```python
from build123d import *

# Parameters (mm, degrees)
F1_DEPTH = 12.7
F3_DEPTH = 25.401
F5_DEPTH = 25.4


with BuildPart() as f1:
    # F0 (on Front) → F1 (new body, symmetric)
    with BuildSketch(Plane.XZ):
        with BuildLine():
            Line((76.2, -76.2), (76.2, 0))
            Line((76.2, 0), (76.2, 76.2))
            Line((76.2, 76.2), (54.9515881949, 76.2))
            ThreePointArc((54.9515881949, 76.2), (49.567872747, 74.095124986), (47.0394765128, 68.8968461044))
            Line((47.0394765128, 68.8968461044), (44.6467865895, 39.0531538956))
            ThreePointArc((44.6467865895, 39.0531538956), (42.1183903553, 33.854875014), (36.7346749074, 31.75))
            Line((36.7346749074, 31.75), (-76.2, 31.75))
            Line((-76.2, 31.75), (-76.2, 0))
            Line((-76.2, 0), (-76.2, -31.75))
            Line((-76.2, -31.75), (36.7346749074, -31.75))
            ThreePointArc((36.7346749074, -31.75), (42.1183903553, -33.854875014), (44.6467865895, -39.0531538956))
            Line((44.6467865895, -39.0531538956), (47.0394765128, -68.8968461044))
            ThreePointArc((47.0394765128, -68.8968461044), (49.567872747, -74.095124986), (54.9515881949, -76.2))
            Line((54.9515881949, -76.2), (76.2, -76.2))
        make_face()
    extrude(amount=F1_DEPTH, both=True)

    # F2 (on face) → F3 (cut, through all)
    with BuildSketch(Plane.XZ.offset(12.7)):
        with BuildLine():
            ThreePointArc((-65.0875, 0), (-67.4123399243, 5.6126600757), (-73.025, 7.9375))
            Line((-73.025, 7.9375), (-76.2, 7.9375))
            Line((-76.2, 7.9375), (-76.2, -7.9375))
            Line((-76.2, -7.9375), (-73.025, -7.9375))
            ThreePointArc((-73.025, -7.9375), (-67.4123399243, -5.6126600757), (-65.0875, 0))
        make_face()
    extrude(amount=-F3_DEPTH, mode=Mode.SUBTRACT)

    # F4 (on face) → F5 (cut)
    with BuildSketch(Plane.XZ.offset(12.7)):
        with BuildLine():
            ThreePointArc((-25.4, -12.7), (-25.4475770151, -11.9241362755), (-25.5895951241, -11.159898781))
            ThreePointArc((-25.5895951241, -11.159898781), (-33.290101219, -6.5395951241), (-37.9104048759, -14.240101219))
            ThreePointArc((-37.9104048759, -14.240101219), (-30.9741362755, -19.0024229849), (-25.4, -12.7))
        make_face()
        with BuildLine():
            ThreePointArc((-31.9395951241, 14.240101219), (-31.7975770151, 13.4758637245), (-31.75, 12.7))
            ThreePointArc((-31.75, 12.7), (-37.3241362755, 6.3975770151), (-44.2604048759, 11.159898781))
            Line((-44.2604048759, 11.159898781), (-37.9104048759, -14.240101219))
            ThreePointArc((-37.9104048759, -14.240101219), (-33.290101219, -6.5395951241), (-25.5895951241, -11.159898781))
            Line((-25.5895951241, -11.159898781), (-31.9395951241, 14.240101219))
        make_face()
        with BuildLine():
            ThreePointArc((-44.2604048759, 11.159898781), (-37.3241362755, 6.3975770151), (-31.75, 12.7))
            ThreePointArc((-31.75, 12.7), (-31.7975770151, 13.4758637245), (-31.9395951241, 14.240101219))
            ThreePointArc((-31.9395951241, 14.240101219), (-39.640101219, 18.8604048759), (-44.2604048759, 11.159898781))
        make_face()
        with BuildLine():
            Line((-55.5874992575, -31.75), (-55.5874992575, -24.8370918305))
            ThreePointArc((-55.5874992575, -24.8370918305), (-62.0395651932, -19.0512714315), (-68.2549589201, -25.0906218393))
            Line((-68.2549589201, -25.0906218393), (-68.2549589201, -31.75))
            Line((-68.2549589201, -31.75), (-55.5874992575, -31.75))
        make_face()
    extrude(amount=-F5_DEPTH, mode=Mode.SUBTRACT)


solid = f1.part
```
Input: part model. Units: mm. Frame: model coordinates. A direction names the side the tool comes from. Coordinates: 2 decimals unless noted, no trailing zeros. Write each loop counter-clockwise with the first axis right and the second up, starting at its lowest first coordinate (ties: lowest second). Pieces come first, ordered by that corner, then holes. Notation, with made-up numbers: (-12, 35) -> (8, 35) arc R28 cw to (8, 73) -> close; hole circle Ø2 at (18, 66). An arc over 180 degrees is marked (long way). Answer as a JSON object with one key per item and string values.
1. Section B-B on x = 24. Return the cut outline in (y, z).
Result set:
{"outline": "(-12.7, -31.75) -> (12.7, -31.75) -> (12.7, 31.75) -> (-12.7, 31.75) -> close"}
2. Material intervals for line 1 (X direction, y = 1, z = -28.5); line 2 (Z direction, x = 16.5, y = 4.25); line 3 (X direction, y = 4.75, z = 6), sorted ascending. Write a range as from..to.
Result set:
{"line 1": "x = -76.2..-68.25, -55.59..76.2", "line 2": "z = -31.75..31.75", "line 3": "x = -67.83..-42.97, -29.88..76.2"}
3. Mould query, pull axis X, two halves, no side actions, for faces 6 (the face through (16, -12.7, 1)), 7 (the face through (-55.587, 0, -28)), 8 (the face through (42.18, -0.18, 33.91)). Classes: released by +X, released by -X, zero draft, split by the parting line, or undercut.
Result set:
{"face 6": "zero draft", "face 7": "undercut", "face 8": "released by -X"}
4. Access query for faces 1 (the face through (-76.2, 0, 20)), 2 (the face through (-68.255, 0, -28)), 3 (the face through (-10, 0, -31.75)), 4 (the face through (-41.13, -0.18, -1.36)), 5 (the face through (-19, 0, 31.75)). Directions: +Z, -Z, +X, -X, +Y, -Y. A direction counts if a zero-diameter tool reaches every point of the face in a straight line with its end or side. Return the directions, or none.
Result set:
{"face 1": "+Z, -Z, -X, +Y, -Y", "face 2": "-Z, +Y, -Y", "face 3": "-Z, -X, +Y, -Y", "face 4": "+Y, -Y", "face 5": "+Z, -X, +Y, -Y"}
5. Section C-C on z = 51. Return the cut outline in (x, y), then the cut area to 3 significant figures.
Result set:
{"outline": "(45.6, -12.7) -> (76.2, -12.7) -> (76.2, 12.7) -> (45.6, 12.7) -> close", "area": "777 mm2"}
6. First-contact query: P1, Ø4, axis at x = 52.5, y = 7.5, coming from the +Z side; P2, Ø5, axis at x = 11.5, y = 5.5, coming from the +Z side; P3, Ø3.5, axis at x = -75, y = 6.5, coming from the -Z side. Flat tips, straight axial feed; report the tip coordinate or a pass-through.
Result set:
{"P1": "stops at z = 76.19", "P2": "stops at z = 31.75", "P3": "stops at z = -31.75"}
